Build history of the part. All positions in model axes, mm. Face numbers are marked on the shaded views. Round coordinates to 2 decimals unless told otherwise and drop trailing zeros. Loops run counter-clockwise (first coordinate to the right, second up) from the corner with the lowest first, then second, coordinate; pieces in that order, holes last. Notation, with made-up numbers: (40.25, -19) -> (93.25, -19) arc R16 ccw to (93.25, -2) -> close; hole circle Ø9 at (-22.5, 23.25). An arc over 180 degrees is marked (long way). Put each result on its own line as item: value. Start each with the question number.
Item 1: Flat gauge pins, fed straight in: pin 1 Ø10 at (y, z) = (-15.5, 10) entering from -X; pin 2 Ø6 at (x, y) = (-35.65, -3.22) entering from +Z; pin 3 Ø5 at (x, z) = (-33.65, 16.5) entering from +Y. Where does each tip first touch, or does it go through?
Item 2: Cut at D-D, the plane z = 16.5. List the corners of the cut face in (x, y), plus the area to 3 significant figures.
Item 3: Drill centre lines: probe 1 along Y at (x, z) = (-35.65, 2.3); probe 2 along Y at (x, z) = (-22, 16.25); probe 3 along Z at (x, y) = (39, -23). Where is each one in solid material? Low to high. Write a range as [from, to].
Item 4: Pull direction Y, two halves, no side cores. Call the marked faces 1, 2 and 3: +Y half, -Y half, draft (parallel to the pull), parting line (faces both ways), or undercut.
Item 5: Cut at B-B, the plane z = 24.5. List the corners of the cut face in (x, y), plus the area to 3 significant figures.
Item 6: Cut at A-A, the plane y = -25. List the corners of the cut face in (x, z).
Item 7: Cut at C-C, the plane y = -10.5. List the corners of the cut face in (x, z).
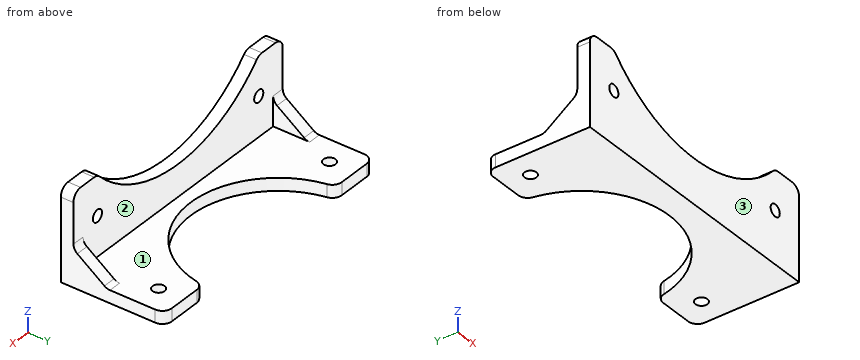
```python
from build123d import *

# Parameters (mm, degrees)
SKETCH1_R      = 1.9
EXTRUDE1_DEPTH = 4
SKETCH2_R      = 1.9
EXTRUDE2_DEPTH = 4
EXTRUDE3_DEPTH = 4
FILLET1_R      = 3


with BuildPart() as part:
    # Sketch1 → Extrude1 (new body)
    with BuildSketch(Plane.XY):
        with BuildLine():
            Line((-43.65, 4.783810266), (-27.65, 4.783810266))
            ThreePointArc((-27.65, 4.783810266), (0, -20.116189734), (27.65, 4.783810266))
            Line((27.65, 4.783810266), (43.65, 4.783810266))
            Line((43.65, 4.783810266), (43.65, -28.116189734))
            Line((43.65, -28.116189734), (-43.65, -28.116189734))
            Line((-43.65, -28.116189734), (-43.65, 4.783810266))
        make_face()
        with Locations((-35.65, -3.216189734)):
            Circle(SKETCH1_R, mode=Mode.SUBTRACT)
        with Locations((35.65, -3.216189734)):
            Circle(SKETCH1_R, mode=Mode.SUBTRACT)
    extrude(amount=EXTRUDE1_DEPTH)



with BuildPart() as body_2:
    # Sketch2 → Extrude2 (new body)
    with BuildSketch(Plane.XZ.offset(28.116189734)):
        with BuildLine():
            Line((-33.65, 29), (-43.65, 29))
            Line((-43.65, 29), (-43.65, 4))
            Line((-43.65, 4), (43.65, 4))
            Line((43.65, 4), (43.65, 29))
            Line((43.65, 29), (33.65, 29))
            ThreePointArc((33.65, 29), (0, 14), (-33.65, 29))
        make_face()
        with Locations((-33.65, 16.5)):
            Circle(SKETCH2_R, mode=Mode.SUBTRACT)
        with Locations((33.65, 16.5)):
            Circle(SKETCH2_R, mode=Mode.SUBTRACT)
    extrude(amount=-EXTRUDE2_DEPTH)


with BuildPart() as part_1:
    add(part.part)

    add(body_2.part)  # Extrude3 merges body 2
    # Sketch3 → Extrude3 (add)
    with BuildSketch(Plane(origin=(43.65, 0, 0), x_dir=(0, 0, -1), z_dir=(1, 0, 0))):
        Polygon((-4, -24.116189734), (-11.756042517, -24.116189734), (-4, -13.510964822), align=None)
    extrude3 = extrude(amount=-EXTRUDE3_DEPTH)

    # Mirror1: Extrude3 across plane
    add(extrude3.mirror(Plane(origin=(0, 0, 0), x_dir=(0, 0, 1), z_dir=(1, 0, 0))))

    # Fillet1
    fillet1_edges = [part_1.edges().sort_by_distance(p)[0] for p in [
        (-43.65, 4.783810266, 2),
        (-27.65, 4.783810266, 2),
        (27.65, 4.783810266, 2),
        (43.65, 4.783810266, 2),
        (41.65, -13.510964822, 4),
        (41.65, -24.116189734, 11.756042517),
        (-33.65, -26.116189734, 29),
        (33.65, -26.116189734, 29),
        (43.65, -26.116189734, 29),
        (-43.65, -26.116189734, 29),
        (-41.65, -13.510964822, 4),
        (-41.65, -24.116189734, 11.756042517),
    ]]
    fillet(fillet1_edges, radius=FILLET1_R)


solid = part_1.part
```
Reply:
1. pin 1: stops at x = -43.65
1. pin 2: stops at z = 4
1. pin 3: stops at y = -24.12
2. outline: (-43.65, -28.12) -> (-35.55, -28.12) -> (-35.55, -24.12) -> (-43.65, -24.12) -> close; (-31.75, -28.12) -> (-14.83, -28.12) -> (-14.83, -24.12) -> (-31.75, -24.12) -> close; (14.83, -28.12) -> (31.75, -28.12) -> (31.75, -24.12) -> (14.83, -24.12) -> close; (35.55, -28.12) -> (43.65, -28.12) -> (43.65, -24.12) -> (35.55, -24.12) -> close
2. area: 200 mm^2
3. probe 1: y = [-28.12, -5.12], [-1.32, 4.78]
3. probe 2: y = [-28.12, -24.12]
3. probe 3: z = [0, 4]
4. face 1: draft
4. face 2: +Y half
4. face 3: -Y half
5. outline: (-43.65, -28.12) -> (-28.98, -28.12) -> (-28.98, -24.12) -> (-43.65, -24.12) -> close; (28.98, -28.12) -> (43.65, -28.12) -> (43.65, -24.12) -> (28.98, -24.12) -> close
5. area: 117 mm^2
6. outline: (-43.65, 0) -> (43.65, 0) -> (43.65, 26) arc R3 ccw to (40.65, 29) -> (34.96, 29) arc R3 ccw to (32.79, 28.07) arc R45.24 cw to (-32.79, 28.07) arc R3 ccw to (-34.96, 29) -> (-40.65, 29) arc R3 ccw to (-43.65, 26) -> close; hole circle Ø3.8 at (-33.65, 16.5); hole circle Ø3.8 at (33.65, 16.5)
7. outline: (-43.65, 0) -> (-21.03, 0) -> (-21.03, 4) -> (-43.65, 4) -> close; (21.03, 0) -> (43.65, 0) -> (43.65, 4) -> (21.03, 4) -> close
